Read the model definition and answer for the solid it produces. Units are mm, in the model's axes. Face numbers are marked on the shaded views. A direction names the side the tool comes from. Give positions to 0.01 mm unless a question says otherwise; leave off trailing zeros. Loops run counter-clockwise (first coordinate to the right, second up) from the corner with the lowest first, then second, coordinate; pieces in that order, holes last. Notation, with made-up numbers: (-6, 84) - (7, 84) arc R9 ccw to (7, 100) - close; hole circle Ø10 at (10, 15). An arc over 180 degrees is marked (long way). Use a Markdown table: item, result. Add a question column.
Item 1: A cutting plane is placed at A-A (x = 2.5). Determine the outline of the cut face in (y, z), plus the area to 3 significant figures.
Item 2: A cutting plane is placed at B-B (x = -2.25). Determine the outline of the cut face in (y, z).
Item 3: A cutting plane is placed at C-C (x = 7.5). Determine the outline of the cut face in (y, z), plus the area to 3 significant figures.
Item 4: Each of these flat-tipped pins is pushed along its axis until it touches: P1, Ø4, axis at x = 2, y = 9, coming from the -Z side; P2, Ø4, axis at x = -7, y = -1.5, coming from the +Z side; P3, Ø10, axis at x = -1.5, z = 3.5, coming from the -Y side. Where does it stop, or does it pass through?
Item 5: Consider probe 1 along Z at (x, y) = (-8.25, -4.5); probe 2 along Y at (x, z) = (-4.5, 5.5); probe 3 along Z at (x, y) = (-8, -2.5). Determine where each line is inside the solid, lowest interval first. Write a range as [from, to].
Item 6: For a pull along Z with two mould halves and no side action, classify the marked faces 1, 2, 3 and 4 as +Z half, -Z half, draft (parallel to the pull), parting line (faces both ways), or undercut.
Item 7: Which of the six approach directions +Z, -Z, +X, -X, +Y, -Y give full straight-line access (tool end or side, diameter ignored) to the marked faces 5, 6, 7 and 8?
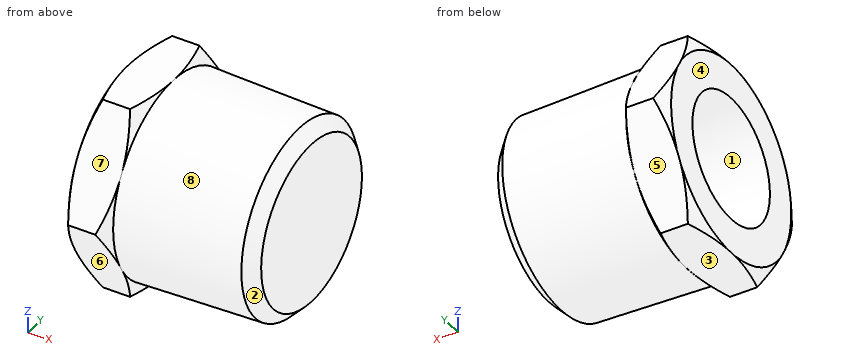
from build123d import *

# Parameters (mm, degrees)
SKETCH2_R          = 10.668
EXTRUDE1_DEPTH     = 15.748
EXTRUDE1_DRAFT     = 1.5
CHAMFER1_SIZE      = 1.366157143
CHAMFER1_SIZE2     = 1.403374095
EXTRUDE2_DEPTH     = 5.08
SKETCH6_R          = 6.858
CUT_EXTRUDE1_DEPTH = 20.983864039
CUT_EXTRUDE1_DRAFT = 1.5
SKETCH12_OUTSIDE_W = 128.474
SKETCH12_OUTSIDE_H = 131.83
SKETCH12_OUTSIDE_R = 11.049
CUT_EXTRUDE6_DEPTH = 27.820778921
CUT_EXTRUDE6_DRAFT = -60
SKETCH13_OUTSIDE_W = 115.58
SKETCH13_OUTSIDE_H = 118.936
SKETCH13_OUTSIDE_R = 11.049
CUT_EXTRUDE7_DEPTH = 24.098660176
CUT_EXTRUDE7_DRAFT = -60


with BuildPart() as part:
    # Sketch2 → Extrude1 (with draft: the straight prism first)
    with BuildSketch(Plane(origin=(10.414, 0, 0), x_dir=(0, 0, -1), z_dir=(1, 0, 0))):
        Circle(SKETCH2_R)
    extrude(amount=-EXTRUDE1_DEPTH)
    # Extrude1: the draft: its side faces are tilted about the plane it starts from
    extrude1_sides = [part.faces().sort_by_distance(p)[0] for p in [
        (2.54, 0, 10.668),
    ]]
    draft(extrude1_sides, Plane(origin=(10.414, 0, 0), x_dir=(0, 0, -1), z_dir=(1, 0, 0)), EXTRUDE1_DRAFT)

    # Chamfer1
    chamfer1_edges = [part.edges().sort_by_distance(p)[0] for p in [
        (10.414, 0, 10.668),
    ]]
    chamfer1_side = [part.faces().sort_by_distance(p)[0] for p in [
        (2.54, 0, 10.874187946),
    ]]
    chamfer(chamfer1_edges, length=CHAMFER1_SIZE, length2=CHAMFER1_SIZE2, reference=chamfer1_side[0])

    # Sketch5 → Extrude2 (add)
    with BuildSketch(Plane.ZY.offset(5.334)):
        Polygon((0, 12.758286249), (-11.049, 6.379143124), (-11.049, -6.379143124), (0, -12.758286249), (11.049, -6.379143124), (11.049, 6.379143124), align=None)
    extrude(amount=EXTRUDE2_DEPTH)


with BuildPart() as cut_extrude1_tool:
    # Sketch6 → Cut-Extrude1 (with draft: the straight prism first)
    with BuildSketch(Plane(origin=(-0.254, 0, 0), x_dir=(0, 0, -1), z_dir=(1, 0, 0))):
        Circle(SKETCH6_R)
    extrude(amount=-CUT_EXTRUDE1_DEPTH)
    # Cut-Extrude1: the draft: its side faces are tilted about the plane it starts from
    cut_extrude1_sides = [cut_extrude1_tool.faces().sort_by_distance(p)[0] for p in [
        (-10.745932019, 0, 6.858),
    ]]
    draft(cut_extrude1_sides, Plane(origin=(-0.254, 0, 0), x_dir=(0, 0, -1), z_dir=(1, 0, 0)), CUT_EXTRUDE1_DRAFT)


with BuildPart() as part_1:
    add(part.part)

    # Cut-Extrude1: cut by cut_extrude1_tool
    add(cut_extrude1_tool.part, mode=Mode.SUBTRACT)


with BuildPart() as cut_extrude6_tool:
    # Sketch12 outside → Cut-Extrude6 (with draft: the straight prism first)
    with BuildSketch(Plane.ZY.offset(10.414)):
        Rectangle(SKETCH12_OUTSIDE_W, SKETCH12_OUTSIDE_H)
        Circle(SKETCH12_OUTSIDE_R, mode=Mode.SUBTRACT)
    extrude(amount=-CUT_EXTRUDE6_DEPTH)
    # Cut-Extrude6: the draft: its side faces are tilted about the plane it starts from
    cut_extrude6_sides = [cut_extrude6_tool.faces().sort_by_distance(p)[0] for p in [
        (3.49638946, -65.915, 0),
        (3.49638946, 0, 64.237),
        (3.49638946, 65.915, 0),
        (3.49638946, 0, -64.237),
        (3.49638946, 0, -11.049),
    ]]
    draft(cut_extrude6_sides, Plane.ZY.offset(10.414), CUT_EXTRUDE6_DRAFT)


with BuildPart() as part_2:
    add(part_1.part)

    # Cut-Extrude6: cut by cut_extrude6_tool
    add(cut_extrude6_tool.part, mode=Mode.SUBTRACT)


with BuildPart() as cut_extrude7_tool:
    # Sketch13 outside → Cut-Extrude7 (with draft: the straight prism first)
    with BuildSketch(Plane(origin=(-5.334, 0, 0), x_dir=(0, 0, -1), z_dir=(1, 0, 0))):
        Rectangle(SKETCH13_OUTSIDE_W, SKETCH13_OUTSIDE_H)
        Circle(SKETCH13_OUTSIDE_R, mode=Mode.SUBTRACT)
    extrude(amount=-CUT_EXTRUDE7_DEPTH)
    # Cut-Extrude7: the draft: its side faces are tilted about the plane it starts from
    cut_extrude7_sides = [cut_extrude7_tool.faces().sort_by_distance(p)[0] for p in [
        (-17.383330088, -59.468, 0),
        (-17.383330088, 0, -57.79),
        (-17.383330088, 59.468, 0),
        (-17.383330088, 0, 57.79),
        (-17.383330088, 0, 11.049),
    ]]
    draft(cut_extrude7_sides, Plane(origin=(-5.334, 0, 0), x_dir=(0, 0, -1), z_dir=(1, 0, 0)), CUT_EXTRUDE7_DRAFT)


with BuildPart() as part_3:
    add(part_2.part)

    # Cut-Extrude7: cut by cut_extrude7_tool
    add(cut_extrude7_tool.part, mode=Mode.SUBTRACT)


solid = part_3.part
Geometry says:
| question | item | result |
|---|---|---|
| 1 | outline | circle Ø21.75 at (0, 0) |
| 1 | area | 372 mm² |
| 2 | outline | circle Ø22 at (0, 0); hole circle Ø13.82 at (0, 0) |
| 3 | outline | circle Ø21.49 at (0, 0) |
| 3 | area | 363 mm² |
| 4 | P1 | z = -8.34 |
| 4 | P2 | z = 11.07 |
| 4 | P3 | y = -12.05 |
| 5 | probe 1 | [-11.05, -5.45], [5.45, 11.05] |
| 5 | probe 2 | [-9.59, -4.28], [4.28, 9.59] |
| 5 | probe 3 | [-11.05, -6.6], [6.6, 11.05] |
| 6 | face 1 | undercut |
| 6 | face 2 | parting line |
| 6 | face 3 | -Z half |
| 6 | face 4 | draft |
| 7 | face 5 | -Z, -X, +Y |
| 7 | face 6 | -Z, -X, -Y |
| 7 | face 7 | +Z, -X, -Y |
| 7 | face 8 | +X |
